The listing builds one solid part. Answer for the finished solid, in the listing's coordinates (mm). A direction names the side the tool comes from. Round coordinates to 2 decimals unless told otherwise and drop trailing zeros. Loops run counter-clockwise (first coordinate to the right, second up) from the corner with the lowest first, then second, coordinate; pieces in that order, holes last. Notation, with made-up numbers: (73.25, -35.5) - (78.25, -35.5) arc R21 ccw to (78.25, -5.5) - close; hole circle Ø11 at (-32.5, 61). An arc over 180 degrees is marked (long way). Write item = value, one per line. Start each with the question number.
1) A tool of negligible diameter and unlimited length cuts with its end or side. For faces 4 (the flat face through (10, 5, 0)), 5 (the flat face through (11, -6, 3.59)), 6 (the flat face through (0, -2, -2)), 7 (the flat face through (11, 6, -3.59)), from which of +Z, -Z, +X, -X, +Y, -Y can it reach the whole face along a straight path? Write none if from no direction.
2) For a pull along Y with two mould halves and no side action, classify faces 1 (the flat face through (6, 0, 0)), 2 (the cylindrical face through (13.744, -6.233, 0.098)), 3 (the cylindrical face through (-4.93, -2.44, -0.54)) as released by +Y, released by -Y, zero draft, split by the parting line, or undercut.
3) Section B-B, the plane x = 6.75 is taken. Determine the outline of the cut face in (y, z).
4) Given pin 1 Ø0.5 at (x, y) = (10.5, 6) entering from -Z; pin 2 Ø1 at (x, z) = (-7, -1) entering from +Y; pin 3 Ø3 at (x, y) = (1, 1.5) entering from +Z; pin 4 Ø1.5 at (x, z) = (-5.5, 5) entering from +Y, each flat-ended and moving along its own axis, determine where each tip first touches the part or whether it passes through.
5) Section D-D, the plane z = -4.5 is taken. Determine the outline of the cut face in (x, y), and give its area (3 significant figures).
6) Section A-A, the plane y = 0 is taken. Determine the outline of the cut face in (x, z), and give its area (3 significant figures).
7) Section C-C, the plane z = 0 is taken. Give the number of separate pieces and of enclosed holes in the cut face, and give its area (4 significant figures).
8) Straight lines are drawn through the part: line 1 along X through (y, z) = (6.7, 0); line 2 along X through (y, z) = (-1, -4.25); line 3 along X through (y, z) = (-4.5, -4.5). For each, find the intervals that lie inside material, in ascending order.
from build123d import *

# Parameters (mm, degrees)
SKETCH1_R               = 5
BOSS_EXTRUDE1_DEPTH     = 4
SKETCH2_R               = 7.5
BOSS_EXTRUDE2_DEPTH     = 2
BOSS_EXTRUDE3_DEPTH     = 10
CUT_EXTRUDE1_DEPTH      = 22.644860822
CUT_EXTRUDE1_DEPTH_BACK = 22.644860822
CUT_EXTRUDE2_DEPTH      = 22.350878369
CUT_EXTRUDE2_DEPTH_BACK = 22.350878369
SKETCH5_R               = 0.75
SKETCH6_R               = 2.5
BOSS_EXTRUDE4_DEPTH     = 10


with BuildPart() as part:
    # Sketch1 → Boss-Extrude1 (new body)
    with BuildSketch(Plane(origin=(0, 0, 0), x_dir=(0, 0, -1), z_dir=(1, 0, 0))):
        Circle(SKETCH1_R)
    extrude(amount=BOSS_EXTRUDE1_DEPTH)

    # Sketch2 → Boss-Extrude2 (add)
    with BuildSketch(Plane(origin=(4, 0, 0), x_dir=(0, 0, -1), z_dir=(1, 0, 0))):
        Circle(SKETCH2_R)
    extrude(amount=BOSS_EXTRUDE2_DEPTH)

    # Sketch3 → Boss-Extrude3 (add)
    with BuildSketch(Plane(origin=(6, 0, 0), x_dir=(0, 0, -1), z_dir=(1, 0, 0))):
        with BuildLine():
            ThreePointArc((5.590169944, 5), (0, 7.5), (-5.590169944, 5))
            Line((-5.590169944, 5), (-4.898979486, 5))
            Line((-4.898979486, 5), (4.898979486, 5))
            Line((4.898979486, 5), (5.590169944, 5))
        make_face()
        with BuildLine():
            Line((-4.898979486, -5), (-5.590169944, -5))
            ThreePointArc((-5.590169944, -5), (0, -7.5), (5.590169944, -5))
            Line((5.590169944, -5), (4.898979486, -5))
            Line((4.898979486, -5), (-4.898979486, -5))
        make_face()
    extrude(amount=BOSS_EXTRUDE3_DEPTH)

    # Sketch4 → Cut-Extrude1 (cut, two sides: drawn at the far end of the back side and taken through both)
    with BuildSketch(Plane.XZ.offset(-5).offset(-CUT_EXTRUDE1_DEPTH_BACK)):
        with BuildLine():
            Line((6, 5.590169944), (16, 5.590169944))
            Line((16, 5.590169944), (16, -5.590169944))
            Line((16, -5.590169944), (6, -5.590169944))
            Line((6, -5.590169944), (9.640400827, -3.590169944))
            Line((9.640400827, -3.590169944), (12.640400827, -3.590169944))
            add(Edge.make_bspline(
                [(12.640400827, -3.590169944), (15.280133609, -2.393446629), (15.919866391, 0), (15.280133609, 2.393446629), (12.640400827, 3.590169944)],
                knots=[0.178885438, 0.178885438, 0.178885438, 0.178885438, 0.5, 0.821114562, 0.821114562, 0.821114562, 0.821114562], degree=3))
            Line((12.640400827, 3.590169944), (9.640400827, 3.590169944))
            Line((9.640400827, 3.590169944), (6, 5.590169944))
        make_face()
    extrude(amount=CUT_EXTRUDE1_DEPTH + CUT_EXTRUDE1_DEPTH_BACK, mode=Mode.SUBTRACT)

    # Sketch5 → Cut-Extrude2 (cut, two sides: drawn at the far end of the back side and taken through both)
    with BuildSketch(Plane.XZ.offset(-5).offset(-CUT_EXTRUDE2_DEPTH_BACK)):
        with Locations(Location((13, 0, 0), (0, 0, 270))):
            Circle(SKETCH5_R)
    extrude(amount=CUT_EXTRUDE2_DEPTH + CUT_EXTRUDE2_DEPTH_BACK, mode=Mode.SUBTRACT)

    # Sketch6 → Boss-Extrude4 (add)
    with BuildSketch(Plane.ZY):
        Circle(SKETCH6_R)
    extrude(amount=BOSS_EXTRUDE4_DEPTH)


solid = part.part
Geometry check:
q1.face_4 = +Z, -Z, +X
q1.face_5 = +Z, +X, +Y, -Y
q1.face_6 = -X
q1.face_7 = -Z, +X, +Y, -Y
q2.face_1 = undercut
q2.face_2 = zero draft
q2.face_3 = split by the parting line
q3.outline = (-5.43, -5.18) - (-5, -5.18) - (-5, 5.18) - (-5.43, 5.18) arc R7.5 ccw to start; (5, -5.18) - (5.43, -5.18) arc R7.5 ccw to (5.43, 5.18) - (5, 5.18) - close
q4.pin_1 = -3.59
q4.pin_2 = 2.45
q4.pin_3 = 5
q4.pin_4 = through
q5.outline = (0, -2.18) - (4, -2.18) - (4, -6) - (7.98, -6) - (7.98, -5) - (6, -5) - (6, 5) - (7.98, 5) - (7.98, 6) - (4, 6) - (4, 2.18) - (0, 2.18) - close
q5.area = 45.4 mm2
q6.outline = (-10, -2.5) - (0, -2.5) - (0, -5) - (4, -5) - (4, -7.5) - (6, -7.5) - (6, 7.5) - (4, 7.5) - (4, 5) - (0, 5) - (0, 2.5) - (-10, 2.5) - close
q6.area = 120 mm2
q7.separate_pieces = 3
q7.enclosed_holes = 0
q7.area = 160.5 mm2
q8.line_1 = 4 to 12.25, 13.75 to 15.6
q8.line_2 = 0 to 6
q8.line_3 = 4 to 6
